Autodesk Inventor part; units mm, degrees
ref_plane "YZ Plane" through (0, 0, 0) normal (1, 0, 0) x (0, 1, 0)
ref_plane "XZ Plane" through (0, 0, 0) normal (0, 1, 0) x (-1, 0, 0)
ref_plane "XY Plane" through (0, 0, 0) normal (0, 0, 1) x (1, 0, 0)
sketch "Sketch1" plane through (0, 0, 0) normal (0, 0, 1) x (1, 0, 0)
  line L0 (0, 0) -> (-375, 0)
  line L1 (-375, 0) -> (-375, -600)
  line L2 (-375, -600) -> (0, -600)
  line L3 (0, -600) -> (0, 0)
  line L4 (-405, 30) -> (30, 30)
  line L5 (30, 30) -> (30, -630)
  line L6 (30, -630) -> (-405, -630)
  line L7 (-405, -630) -> (-405, 30)
  line L8 (-405, -630) -> (-375, -630)
  line L9 (-375, -630) -> (-375, -1270)
  line L10 (-375, -1270) -> (-405, -1270)
  line L11 (-405, -1270) -> (-405, -630)
  line L12 (30, -630) -> (0, -630)
  line L13 (0, -630) -> (0, -1270)
  line L14 (0, -1270) -> (30, -1270)
  line L15 (30, -1270) -> (30, -630)
  line L16 (-375, -1270) -> (0, -1270)
  line L17 (0, -1270) -> (0, -1240)
  line L18 (0, -1240) -> (-375, -1240)
  line L19 (-375, -1240) -> (-375, -1270)
  dimension "d0" = 375
  dimension "d1" = 600
  dimension "d2" = 30
  dimension "d3" = 30
  dimension "d4" = 30
  dimension "d5" = 30
  dimension "d38" = 30
  dimension "d39" = 640
  dimension "d40" = 30
  dimension "d41" = 640
  dimension "d42" = 30
extrude "Extrusion1" add sketch "Sketch1" along normal blind 30 contours L4 L5 L6 L7
sketch "Sketch2" plane through (0, 0, 0) normal (0, 0, -1) x (-1, 0, 0)
  line L0 (375, -600) -> (375, 0)
  line L1 (375, -450) -> (0, -450)
  line L2 (0, -450) -> (0, -410)
  line L3 (0, -410) -> (375, -410)
  line L4 (375, -410) -> (375, -450)
  line L5 (0, -600) -> (375, -600)
  line L6 (202.5, -600) -> (202.5, -450)
  line L7 (172.5, -600) -> (172.5, -450)
  point P0 (0, 0)
  dimension "d8" = 375
  dimension "d9" = 40
  dimension "d10" = 150
extrude "Extrusion2" add sketch "Sketch2" against normal blind 30 contours L1 L2 L3 L0 | L5 L7 L1 L6
sketch "Sketch3" plane through (0, 0, 30) normal (0, 0, 1) x (1, 0, 0)
  line L0 (12.5, -490) -> (17.5, -490)
  line L1 (17.5, -490) -> (17.5, -200)
  line L2 (17.5, -200) -> (12.5, -200)
  line L3 (12.5, -200) -> (12.5, -490)
  line L4 (0, -410) -> (-375, -410)
  line L5 (-392.5, -490) -> (-387.5, -490)
  line L6 (-387.5, -490) -> (-387.5, -200)
  line L7 (-387.5, -200) -> (-392.5, -200)
  line L8 (-392.5, -200) -> (-392.5, -490)
  line L9 (0, -600) -> (-172.5, -600)
  point P0 (0, 0)
  dimension "d13" = 5
  dimension "d14" = 290
  dimension "d18" = 405
  dimension "d37" = 110
extrude "Extrusion3" add sketch "Sketch3" along normal blind 80
sketch "Sketch4" plane through (30, -630, 0) normal (1, 0, 0) x (0, 0, -1)
  line L0 (-30, 0) -> (-30, 660)
  line L1 (-30, 660) -> (-657.8518, 828.2324)
  line L2 (-30, 660) -> (620, 660) construction
  line L3 (-657.8518, 828.2324) -> (-665.6164, 799.2546)
  line L4 (-665.6164, 799.2546) -> (-30, 628.9417)
  point P0 (0, 630)
  dimension "d25" = 650
  dimension "d26" = 165
  dimension "d27" = 30
  dimension "d28" = 270
extrude "Extrusion4" add sketch "Sketch4" against normal blind 30
pattern_linear "Rectangular Pattern1" count 2 spacing 405 along (-1, 0, 0) of "Extrusion4"
sketch "Sketch5" plane through (-375, 0, 30) normal (1, 0, 0) x (0, 0, -1)
  line L0 (-635.6164, 169.2546) -> (-627.8518, 198.2324)
  line L1 (0, -1.0583) -> (-635.6164, 169.2546)
  line L2 (-627.8518, 198.2324) -> (-635.6164, 169.2546)
  line L3 (-635.6164, 169.2546) -> (-606.6386, 161.49)
  line L4 (-606.6386, 161.49) -> (-598.874, 190.4678)
  line L5 (-627.8518, 198.2324) -> (0, 30)
  line L6 (-627.8518, 198.2324) -> (-598.874, 190.4678)
  point P0 (30, 0)
  dimension "d34" = 30
extrude "Extrusion5" add sketch "Sketch5" along normal up to surface (375 mm away)
sketch "Sketch6" plane through (0, 0, 0) normal (0, 0, -1) x (-1, 0, 0)
  line L0 (0, -630) -> (0, -1270)
  line L1 (0, -1270) -> (-30, -1270)
  line L2 (-30, -1270) -> (-30, -630)
  line L3 (375, -630) -> (375, -1270)
  line L4 (375, -1270) -> (405, -1270)
  line L5 (405, -1270) -> (405, -630)
  line L6 (0, -1270) -> (375, -1270)
  line L7 (375, -1270) -> (375, -1240)
  line L8 (375, -1240) -> (0, -1240)
  line L9 (0, -1240) -> (0, -1270)
  line L10 (405, -1.0583) -> (405, -630)
  line L11 (-30, -630) -> (-30, -1.0583)
  line L12 (405, -630) -> (375, -630)
  line L13 (405, -630) -> (-30, -630)
  line L14 (0, -630) -> (-30, -630)
  point P0 (0, 0)
  dimension "d43" = 30
  dimension "d44" = 640
  dimension "d45" = 30
  dimension "d46" = 640
  dimension "d47" = 30
  dimension "d48" = 0
  dimension "d49" = 0
extrude "Extrusion6" add sketch "Sketch6" against normal blind 30 contours L0 L1 L2 L13 | L8 L3 L6 L0 | L12 L5 L4 L3
sketch "Sketch7" plane through (0, 0, 0) normal (0, 0, -1) x (-1, 0, 0)
  circle A0 centre (187.5, -430) radius 40
  point P0 (0, 0)
  dimension "d52" = 80
extrude "Extrusion7" add sketch "Sketch7" along normal blind 5 and the other way blind 5
sketch "Sketch8" plane through (30, -1270, 0) normal (1, 0, 0) x (0, 0, -1)
  line L0 (0, 0) -> (-30, 0)
  line L1 (-30, 0) -> (-311.9078, 102.606)
  line L2 (-30, 0) -> (270, 0) construction
  line L3 (-311.9078, 102.606) -> (-301.6472, 130.7968)
  line L4 (-301.6472, 130.7968) -> (-30, 31.9253)
  line L5 (-30, 640) -> (-30, 30)
  line L6 (-30, 31.9253) -> (-30, 0)
  point P0 (0, 1270)
  dimension "d55" = 300
  dimension "d56" = 160
  dimension "d57" = 30
  dimension "d58" = 90
extrude "Extrusion8" add sketch "Sketch8" against normal blind 30
pattern_linear "Rectangular Pattern2" count 2 spacing 405 along (-1, 0, 0) of "Extrusion8"
sketch "Sketch9" plane through (0, -1240, 0) normal (-1, 0, 0) x (0, 0, 1)
  line L0 (311.9078, 72.606) -> (301.6472, 100.7968)
  line L1 (311.9078, 72.606) -> (301.6472, 100.7968)
  line L2 (301.6472, 100.7968) -> (273.4564, 90.5362)
  line L3 (30, 1.9253) -> (301.6472, 100.7968)
  line L4 (273.4564, 90.5362) -> (283.717, 62.3454)
  line L5 (30, -30) -> (311.9078, 72.606)
  line L6 (283.717, 62.3454) -> (311.9078, 72.606)
  point P0 (0, 1240)
  dimension "d64" = 30
extrude "Extrusion9" add sketch "Sketch9" along normal up to surface (375 mm away)
sketch "Sketch10" plane through (0, 0, 30) normal (0, 0, 1) x (1, 0, 0)
  line L0 (-405, -1238.0747) -> (-375, -1238.0747)
  line L1 (-405, -1238.0747) -> (30, -1238.0747)
  line L2 (30, -1238.0747) -> (30, -598.0747)
  line L3 (30, -598.0747) -> (-405, -598.0747)
  line L4 (-405, -598.0747) -> (-405, -1238.0747)
  point P0 (0, 0)
  dimension "d67" = 435
  dimension "d68" = 640
extrude "Extrusion10" add sketch "Sketch10" along normal blind 2
sketch "Sketch11" plane through (0, 0, 32) normal (0, 0, 1) x (1, 0, 0)
  line L0 (30, -648.0747) -> (0, -648.0747)
  line L1 (0, -648.0747) -> (0, -678.0747)
  line L2 (0, -678.0747) -> (30, -678.0747)
  line L3 (30, -678.0747) -> (30, -648.0747)
  line L4 (30, -598.0747) -> (-405, -598.0747)
  point P0 (0, 0)
  dimension "d71" = 30
  dimension "d72" = 30
  dimension "d73" = 50
extrude "Extrusion11" add sketch "Sketch11" along normal blind 350
pattern_linear "Rectangular Pattern3" count 2 spacing 220 along (0, -1, 0) count 2 spacing 405 along (-1, 0, 0) of "Extrusion11"
sketch "Sketch12" plane through (0, 0, 382) normal (0, 0, 1) x (1, 0, 0)
  line L0 (-405, -868.0747) -> (-405, -898.0747)
  line L1 (-405, -898.0747) -> (-375, -898.0747)
  line L2 (-375, -898.0747) -> (-375, -868.0747)
  line L3 (-375, -868.0747) -> (-405, -868.0747)
  line L4 (-405, -648.0747) -> (-405, -678.0747)
  line L5 (-405, -678.0747) -> (-375, -678.0747)
  line L6 (-375, -678.0747) -> (-375, -648.0747)
  line L7 (-375, -648.0747) -> (-405, -648.0747)
  line L8 (0, -648.0747) -> (0, -678.0747)
  line L9 (0, -678.0747) -> (30, -678.0747)
  line L10 (30, -678.0747) -> (30, -648.0747)
  line L11 (30, -648.0747) -> (0, -648.0747)
  line L12 (0, -868.0747) -> (0, -898.0747)
  line L13 (0, -898.0747) -> (30, -898.0747)
  line L14 (30, -898.0747) -> (30, -868.0747)
  line L15 (30, -868.0747) -> (0, -868.0747)
  line L16 (-405, -898.0747) -> (-375, -898.0747)
  line L17 (-405, -898.0747) -> (30, -898.0747)
  line L18 (30, -898.0747) -> (30, -648.0747)
  line L19 (30, -648.0747) -> (-405, -648.0747)
  line L20 (-405, -648.0747) -> (-405, -898.0747)
  point P0 (0, 0)
  point P1 (0, -898.0747)
  point P2 (30, -868.0747)
  point P3 (30, -678.0747)
  point P4 (0, -648.0747)
extrude "Extrusion12" add sketch "Sketch12" against normal blind 3 contours L20 L5 L6 L19 L8 L9 L18 L15 L12 L17 L2 L3
sketch "Sketch13" plane through (-405, -1270, 0) normal (-1, 0, 0) x (0, 0, 1)
  line L0 (232, 591.9253) -> (202, 591.9253)
  line L1 (202, 591.9253) -> (202, 741.9253)
  line L2 (202, 741.9253) -> (232, 741.9253)
  line L3 (232, 741.9253) -> (232, 591.9253)
  line L4 (32, 591.9253) -> (379, 591.9253)
  line L5 (382, 621.9253) -> (382, 371.9253)
  point P0 (0, 1270)
  dimension "d84" = 30
  dimension "d85" = 150
  dimension "d86" = 0
  dimension "d87" = 150
extrude "Extrusion13" add sketch "Sketch13" along normal blind 30
sketch "Sketch14" plane through (-435, -1270, 0) normal (-1, 0, 0) x (0, 0, 1)
  line L0 (232, 741.9253) -> (202, 741.9253)
  line L1 (232, 741.9253) -> (202, 741.9253)
  line L2 (202, 741.9253) -> (202, 711.9253)
  line L3 (202, 711.9253) -> (232, 711.9253)
  line L4 (232, 711.9253) -> (232, 741.9253)
  point P0 (0, 1270)
  point P1 (202, 741.9253)
  dimension "d90" = 30
  dimension "d91" = 30
extrude "Extrusion14" add sketch "Sketch14" along normal blind 250
sketch "Sketch15" plane through (30, -1270, 0) normal (1, 0, 0) x (0, 0, -1)
  line L0 (-657.8518, 1468.2324) -> (-665.6164, 1439.2546) construction
  circle A0 centre (-661.7341, 1453.7435) radius 7.5 construction
  circle A1 centre (-654.5905, 1451.4588) radius 4
  point P0 (0, 1270)
  dimension "d96" = 15
  dimension "d97" = 8
extrude "Extrusion15" cut sketch "Sketch15" against normal through all
properties part number "rama pod fotel v2"
Work out the finished part from the listing and answer in its coordinate system (mm). A direction names the side the tool comes from. Give positions to 0.01 mm unless a question says otherwise; leave off trailing zeros. Write each loop counter-clockwise with the first axis right and the second up, starting at its lowest first coordinate (ties: lowest second). Pieces come first, ordered by that corner, then holes. Notation, with made-up numbers: (40, 3) - (77, 3) arc R21 ccw to (77, 38) - close; hole circle Ø2 at (-7, 46). An arc over 180 degrees is marked (long way). Use one line per item in the form item = value.
1. Consider L1, parallel to Z at x = -325.5, y = -1008; L2, parallel to X at y = -169.5, z = 27. Determine where each line is inside the solid, lowest interval first.
Filled in:
L1 = 30 to 32
L2 = -405 to -375, 0 to 30
2. A cutting plane is placed at B-B (y = 65.5). Write down the section's boundary in (x, z).
Filled in:
outline = (-405, 162.49) - (-375, 162.49) - (-375, 278.4) - (-405, 278.4) - close; (0, 162.49) - (30, 162.49) - (30, 278.4) - (0, 278.4) - close
3. A cutting plane is placed at A-A (x = -282). State how many separate pieces and enclosed holes the cut face has, and give its area (3 significant figures).
Filled in:
separate_pieces = 7
enclosed_holes = 1
area = 7,680 mm^2
4. Determine the mould class of faces 6 (the face through (-190.5, 183.5, 661.8)), 7 (the face through (-503, -553, 232)), 8 (the face through (-185, -630, 15)) for opening direction Y: released by +Y, released by -Y, zero draft, split by the parting line, or undercut.
Filled in:
face_6 = released by +Y
face_7 = zero draft
face_8 = undercut
5. For faces 1 (the face through (0, -1020, 27)), 2 (the face through (-190.12, 175.78, 632.81)), 3 (the face through (-392.5, -343, 69)), 4 (the face through (12.5, -343, 69)), 5 (the face through (-382, -898.075, 206)), determine the directions among +Z, -Z, +X, -X, +Y, -Y from which every point of the face is accessible in a straight line to the end or side of a thin tool.
Filled in:
face_1 = none
face_2 = -Z, -Y
face_3 = +Z, -X
face_4 = +Z
face_5 = +Z, +X, -X
6. Each of these flat-tipped pins is pushed along its axis until it touches: pin 1 Ø8 at (x, y) = (-438.5, -577) entering from +Z; pin 2 Ø5 at (x, y) = (-159.5, -462.5) entering from +Z; pin 3 Ø5.5 at (x, y) = (15.5, -415) entering from +Z; pin 4 Ø4 at (x, y) = (-367, -687) entering from +Z. Where does it stop, or does it pass through?
Filled in:
pin_1 = 232
pin_2 = through
pin_3 = 110
pin_4 = 382
